Read the model definition and answer for the solid it produces. Units are mm, in the model's axes. A direction names the side the tool comes from. Coordinates: 2 decimals unless noted, no trailing zeros. Order: outer loops, then holes, each group sorted by start corner. A loop starts at its lowest first (then second) coordinate and runs counter-clockwise, first axis right, second up. Notation, with made-up numbers: (74, 15) -> (121, 15) arc R27 ccw to (121, 40) -> close; hole circle Ø10 at (21, -12.75). An arc over 180 degrees is marked (long way). Answer in a Markdown table with one row per item.
from build123d import *

# Parameters (mm, degrees)
F1_DEPTH  = 44
F2_R      = 54
F2_R_2    = 28.575
F3_DEPTH  = 64
F4_W      = 114
F4_H      = 50
F5_DEPTH  = 22
F6_R      = 11.1
F7_DEPTH  = 22.001
F9_DEPTH  = 64.001
F11_DEPTH = 95.001


with BuildPart() as f1:
    # F0 (on Front) → F1 (new body)
    with BuildSketch(Plane.XZ):
        with BuildLine():
            ThreePointArc((35.1425667816, 41), (49.0596504584, 22.5643678594), (54, 0))
            Line((54, 0), (174, 0))
            Line((174, 0), (174, 41))
            Line((174, 41), (35.1425667816, 41))
        make_face()
        with BuildLine():
            Line((174, 0), (54, 0))
            ThreePointArc((54, 0), (49.0596504584, -22.5643678594), (35.1425667816, -41))
            Line((35.1425667816, -41), (174, -41))
            Line((174, -41), (174, 0))
        make_face()
    extrude(amount=F1_DEPTH)

    # F2 (on Front) → F3 (join)
    with BuildSketch(Plane.XZ):
        Circle(F2_R)
        Circle(F2_R_2, mode=Mode.SUBTRACT)
        Circle(F2_R_2)
    extrude(amount=F3_DEPTH)

    # F4 (on face) → F5 (cut)
    with BuildSketch(Plane.XZ.offset(44)):
        with Locations((117, 0)):
            Rectangle(F4_W, F4_H)
    extrude(amount=-F5_DEPTH, mode=Mode.SUBTRACT)

    # F6 (on face) → F7 (cut, through all)
    with BuildSketch(Plane.XZ.offset(22)):
        with BuildLine():
            Line((139, 0), (150.1, 0))
            ThreePointArc((150.1, 0), (139, 11.1), (127.9, 0))
            Line((127.9, 0), (139, 0))
        make_face()
        with BuildLine():
            ThreePointArc((127.9, 0), (139, -11.1), (150.1, 0))
            Line((150.1, 0), (139, 0))
            Line((139, 0), (127.9, 0))
        make_face()
        with Locations((89, 0)):
            Circle(F6_R)
    extrude(amount=-F7_DEPTH, mode=Mode.SUBTRACT)

    # F8 (on face) → F9 (cut, through all)
    with BuildSketch(Plane.XZ.offset(64)):
        with BuildLine():
            ThreePointArc((-28.575, 0), (0, -28.575), (28.575, 0))
            ThreePointArc((28.575, 0), (0, 28.575), (-28.575, 0))
        make_face()
    extrude(amount=-F9_DEPTH, mode=Mode.SUBTRACT)

    # F10 (on face) → F11 (cut, through all)
    with BuildSketch(Plane.XY.offset(41)):
        Polygon((174, -32), (162, -44), (174, -44), align=None)
    extrude(amount=-F11_DEPTH, mode=Mode.SUBTRACT)


solid = f1.part
Q1. The part is cut by section C-C (z = 21). Write down the section's boundary in (x, y), then the cut area to 3 significant figures.
Outcome:
| item | result |
|---|---|
| outline | (-49.75, -64) -> (-19.38, -64) -> (-19.38, 0) -> (-49.75, 0) -> close; (19.38, -64) -> (49.75, -64) -> (49.75, -44) -> (60, -44) -> (60, -22) -> (174, -22) -> (174, 0) -> (19.38, 0) -> close |
| area | 6,850 mm² |
Q2. Given pin 1 (22 mm diameter, centred on x = 125, y = -12, fed in from -Z); pin 2 (24.5 mm diameter, centred on x = 105, z = 7, fed in from -Y); pin 3 (4 mm diameter, centred on y = -50, z = -28, fed in from +X), each flat-ended and moving along its own axis, determine where each tip first touches the part or whether it passes through.
Outcome:
| item | result |
|---|---|
| pin 1 | z = -41 |
| pin 2 | y = -22 |
| pin 3 | x = 47.33 |
Q3. Consider line 1 (Z direction, x = 139, y = -14); line 2 (Y direction, x = 80.5, z = -36.5); line 3 (Z direction, x = -16.5, y = -28.5). Determine where each line is inside the solid, lowest interval first.
Outcome:
| item | result |
|---|---|
| line 1 | -41 to -11.1, 11.1 to 41 |
| line 2 | -44 to 0 |
| line 3 | -51.42 to -23.33, 23.33 to 51.42 |
Q4. For faces 5 (the face through (116, -33, 25)), 6 (the face through (104, -22, -41)), 7 (the face through (58, 0, 1)), determine the directions among +Z, -Z, +X, -X, +Y, -Y from which every point of the face is accessible in a straight line to the end or side of a thin tool.
Outcome:
| item | result |
|---|---|
| face 5 | +X, -Y |
| face 6 | -Z, +X, +Y, -Y |
| face 7 | +Z, -Z, +X, -X, +Y |
Q5. The part is cut by section B-B (y = -17.5). Write down the section's boundary in (x, z) (3 decimals), then the cut area to 3 significant figures.
Outcome:
| item | result |
|---|---|
| outline | (35.143, -41) -> (174, -41) -> (174, 41) -> (35.143, 41) arc R54 ccw (long way) to start; hole circle Ø57.15 at (0, 0); hole circle Ø22.2 at (89, 0); hole circle Ø22.2 at (139, 0) |
| area | 16,100 mm² |
Q6. The part is cut by section D-D (x = 72). Write down the section's boundary in (y, z).
Outcome:
| item | result |
|---|---|
| outline | (-44, -41) -> (0, -41) -> (0, 41) -> (-44, 41) -> (-44, 25) -> (-22, 25) -> (-22, -25) -> (-44, -25) -> close |
Q7. The part is cut by section A-A (x = 139). Write down the section's boundary in (y, z).
Outcome:
| item | result |
|---|---|
| outline | (-44, -41) -> (0, -41) -> (0, -11.1) -> (-22, -11.1) -> (-22, -25) -> (-44, -25) -> close; (-44, 25) -> (-22, 25) -> (-22, 11.1) -> (0, 11.1) -> (0, 41) -> (-44, 41) -> close |
Q8. For a pull along Z with two mould halves and no side action, classify faces 1 (the face through (116, -33, -25)), 2 (the face through (116, -22, 0)), 3 (the face through (106, -22, 41)), 4 (the face through (98, -44, 28)) as pulls with the +Z half, pulls with the -Z half, needs draft (parallel to the pull), parting line crosses it, or undercut.
Outcome:
| item | result |
|---|---|
| face 1 | undercut |
| face 2 | undercut |
| face 3 | pulls with the +Z half |
| face 4 | needs draft |
